Part model, mm, in its own coordinate system. Face numbers are marked on the shaded views. A direction names the side the tool comes from. Give positions to 0.01 mm unless a question says otherwise; leave off trailing zeros. Write each loop counter-clockwise with the first axis right and the second up, starting at its lowest first coordinate (ties: lowest second). Pieces come first, ordered by that corner, then holes. Notation, with made-up numbers: M 85.25,47 L 95.25,47 A21 ccw 95.25,58 Z; hole C 16,0.25 d6. An arc over 180 degrees is marked long. Use CSV: the item, a comma, the result in double quotes. Start each with the question number.
1. Band-saw the part on A-A, the plane x = 0. List the corners of the cut face in (y, z), then the cut area to 3 significant figures.
2. Band-saw the part on C-C, the plane z = 4.5. List the corners of the cut face in (x, y), then the cut area to 3 significant figures.
3. Drill centre lines: line 1 along Z through (x, y) = (-1.25, 2.45); line 2 along Y through (x, z) = (1.95, 4); line 3 along X through (y, z) = (-1.6, 5.25). Where is each one in solid material? Low to high. Write a range as from..to.
4. Drop flat-ended pins along their axis: pin 1 Ø1.5 at (x, y) = (1, 1) entering from -Z; pin 2 Ø2 at (x, y) = (-1.5, -1) entering from +Z; pin 3 Ø1.5 at (x, z) = (2, 3.5) entering from +Y. Give the stop position or say it passes through.
5. Band-saw the part on B-B, the plane y = 1. List the corners of the cut face in (x, z).
6. Band-saw the part on D-D, the plane y = -2.3. List the corners of the cut face in (x, z).
7. 3-axis set-ups, long thin cutter, end or side, ignore diameter. For the marked faces 1 and 2: which of +Z, -Z, +X, -X, +Y, -Y reach the whole face in a straight line?
from build123d import *

# Parameters (mm, degrees)
ESBO_O1_R                = 3
RESSALTO_EXTRUS_O1_DEPTH = 1
CORTE_EXTRUS_O1_DEPTH    = 1


with BuildPart() as part:
    # Esboço1 → Ressalto-extrusão1 (new body)
    with BuildSketch(Plane.XY):
        Circle(ESBO_O1_R)
    extrude(amount=RESSALTO_EXTRUS_O1_DEPTH)

    # Esboço3 → Revolução1 (revolve)
    with BuildSketch(Plane(origin=(0, 0, 0), x_dir=(0, 0, -1), z_dir=(1, 0, 0))):
        with BuildLine():
            Line((-1, 0), (-8.8, 0))
            ThreePointArc((-8.8, 0), (-8.067766953, 1.767766953), (-6.3, 2.5))
            Line((-6.3, 2.5), (-1, 2.5))
            Line((-1, 2.5), (-1, 0))
        make_face()
    revolve(axis=Axis((0, 0, 1), (0, 0, 1)))

    # Esboço4 → Corte-extrusão1 (cut)
    with BuildSketch(Plane(origin=(0, 0, 0), x_dir=(-1, 0, 0), z_dir=(0, 0, -1))):
        with BuildLine():
            Line((2.5, 1.658312395), (2.5, -1.658312395))
            ThreePointArc((2.5, -1.658312395), (3, 0), (2.5, 1.658312395))
        make_face()
    extrude(amount=-CORTE_EXTRUS_O1_DEPTH, mode=Mode.SUBTRACT)


solid = part.part
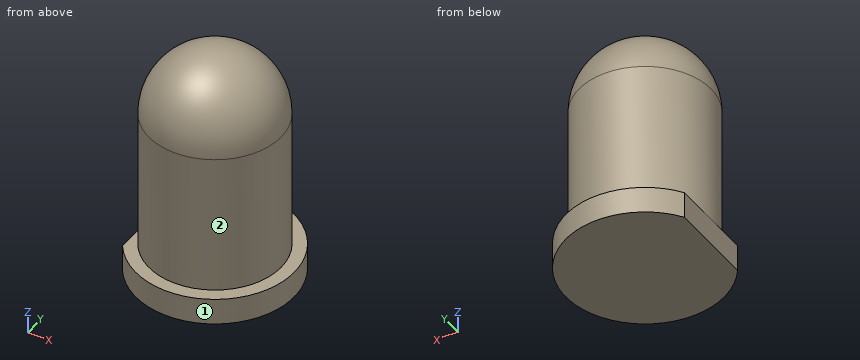
Output:
1,outline,"M -3,0 L 3,0 L 3,1 L 2.5,1 L 2.5,6.3 A2.5 ccw -2.5,6.3 L -2.5,1 L -3,1 Z"
1,area,"42.3 mm²"
2,outline,"C 0,0 d5"
2,area,"19.6 mm²"
3,line 1,"z = 0..1"
3,line 2,"y = -1.56..1.56"
3,line 3,"x = -1.92..1.92"
4,pin 1,"stops at z = 0"
4,pin 2,"stops at z = 8.67"
4,pin 3,"stops at y = 2.17"
5,outline,"M -2.5,0 L 2.83,0 L 2.83,1 L 2.29,1 L 2.29,6.3 A2.29 ccw -2.29,6.3 L -2.29,1 L -2.5,1 Z"
6,outline,"M -1.93,0 L 1.93,0 L 1.93,1 L 0.98,1 L 0.98,6.3 A0.98 ccw -0.98,6.3 L -0.98,1 L -1.93,1 Z"
7,face 1,"+Z, -Z"
7,face 2,"+Z"
